```python
from build123d import *

# Parameters (mm, degrees)
F1_DEPTH = 20
F0_W     = 4
F0_H     = 2.9398608957
F2_DEPTH = 58
F4_DEPTH = 4
F5_DEPTH = 20
F7_DEPTH = 9


# Not quite as in the source:
# - a feature names something its author has since deleted; it is built from what else it names


with BuildPart() as f1:
    # F0 (on Top) → F1 (new body)
    with BuildSketch(Plane.XY):
        with BuildLine():
            Line((0, 13.7), (-25, 13.7))
            Line((-25, 13.7), (-25, -6))
            Line((-25, -6), (-12.3162494291, -6))
            ThreePointArc((-12.3162494291, -6), (-11.6165829744, 7.2625753008), (0, 13.7))
        make_face()
    extrude(amount=F1_DEPTH)



with BuildPart() as f1b:
    # F0 (on Top) → F1, piece 2 (new body)
    with BuildSketch(Plane.XY):
        with BuildLine():
            Line((25, 13.7), (0, 13.7))
            ThreePointArc((0, 13.7), (9.6873629023, 9.6873629023), (13.7, 0))
            ThreePointArc((13.7, 0), (13.3495808395, -3.0787483513), (12.3162494291, -6))
            Line((12.3162494291, -6), (25, -6))
            Line((25, -6), (25, 13.7))
        make_face()
    extrude(amount=F1_DEPTH)


with BuildPart() as f1_1:
    add(f1.part)

    add(f1b.part)  # F2 merges F1b
    # F0 (on Top) → F2 (join)
    with BuildSketch(Plane.XY):
        with BuildLine():
            ThreePointArc((13.7, 0), (9.6873629023, 9.6873629023), (0, 13.7))
            ThreePointArc((0, 13.7), (-11.6165829744, 7.2625753008), (-12.3162494291, -6))
            Line((-12.3162494291, -6), (-7.6216796049, -6))
            ThreePointArc((-7.6216796049, -6), (-3.1748785672, 9.1657048875), (9.7, 0))
            ThreePointArc((9.7, 0), (9.1657048875, -3.1748785672), (7.6216796049, -6))
            Line((7.6216796049, -6), (12.3162494291, -6))
            ThreePointArc((12.3162494291, -6), (13.3495808395, -3.0787483513), (13.7, 0))
        make_face()
        with BuildLine():
            Line((-7.6216796049, -6), (-12.3162494291, -6))
            ThreePointArc((-12.3162494291, -6), (-9.0959869464, -10.244658192), (-4.5, -12.9398608957))
            ThreePointArc((-4.5, -12.9398608957), (-2.5280436601, -13.4647315329), (-0.5, -13.6908728721))
            Line((-0.5, -13.6908728721), (-0.5, -9.6871048306))
            ThreePointArc((-0.5, -9.6871048306), (-4.4597203286, -8.6139941137), (-7.6216796049, -6))
        make_face()
        with BuildLine():
            ThreePointArc((4.5, -12.9398608957), (9.0959869464, -10.244658192), (12.3162494291, -6))
            Line((12.3162494291, -6), (7.6216796049, -6))
            ThreePointArc((7.6216796049, -6), (4.4597203286, -8.6139941137), (0.5, -9.6871048306))
            Line((0.5, -9.6871048306), (0.5, -13.6908728721))
            ThreePointArc((0.5, -13.6908728721), (2.5280436601, -13.4647315329), (4.5, -12.9398608957))
        make_face()
        with Locations((2.5, -15.4699304478)):
            Rectangle(F0_W, F0_H)
        with BuildLine():
            Line((4.5, -14), (4.5, -12.9398608957))
            ThreePointArc((4.5, -12.9398608957), (2.5280436601, -13.4647315329), (0.5, -13.6908728721))
            Line((0.5, -13.6908728721), (0.5, -14))
            Line((0.5, -14), (4.5, -14))
        make_face()
        with BuildLine():
            ThreePointArc((-0.5, -13.6908728721), (-2.5280436601, -13.4647315329), (-4.5, -12.9398608957))
            Line((-4.5, -12.9398608957), (-4.5, -14))
            Line((-4.5, -14), (-0.5, -14))
            Line((-0.5, -14), (-0.5, -13.6908728721))
        make_face()
        with Locations((-2.5, -15.4699304478)):
            Rectangle(F0_W, F0_H)
    extrude(amount=F2_DEPTH)

    # F3 (on face) → F4 (cut)
    with BuildSketch(Plane.XZ.offset(6)):
        with BuildLine():
            ThreePointArc((-21.3581247146, 10), (-18.6581247146, 12.7), (-15.9581247146, 10))
            Line((-15.9581247146, 10), (-13.4831247146, 10))
            ThreePointArc((-13.4831247146, 10), (-18.6581247146, 15.175), (-23.8331247146, 10))
            Line((-23.8331247146, 10), (-21.3581247146, 10))
        make_face()
        with BuildLine():
            Line((-13.4831247146, 10), (-15.9581247146, 10))
            ThreePointArc((-15.9581247146, 10), (-18.6581247146, 7.3), (-21.3581247146, 10))
            Line((-21.3581247146, 10), (-23.8331247146, 10))
            ThreePointArc((-23.8331247146, 10), (-18.6581247146, 4.825), (-13.4831247146, 10))
        make_face()
        with BuildLine():
            ThreePointArc((23.8331247146, 10), (18.6581247146, 15.175), (13.4831247146, 10))
            Line((13.4831247146, 10), (15.9581247146, 10))
            ThreePointArc((15.9581247146, 10), (18.6581247146, 12.7), (21.3581247146, 10))
            Line((21.3581247146, 10), (23.8331247146, 10))
        make_face()
        with BuildLine():
            Line((15.9581247146, 10), (13.4831247146, 10))
            ThreePointArc((13.4831247146, 10), (18.6581247146, 4.825), (23.8331247146, 10))
            Line((23.8331247146, 10), (21.3581247146, 10))
            ThreePointArc((21.3581247146, 10), (18.6581247146, 7.3), (15.9581247146, 10))
        make_face()
    extrude(amount=-F4_DEPTH, mode=Mode.SUBTRACT)

    # F5 (cut): faces of the model
    f5_faces = [f1_1.faces().sort_by_distance(p)[0] for p in [
        (-18.6581247146, -6, 10),
        (18.6581247146, -6, 10),
    ]]
    extrude(f5_faces, amount=-F5_DEPTH, mode=Mode.SUBTRACT)

    # F6 (on face) → F7 (cut)
    with BuildSketch(Plane(origin=(-4.5, 0, 0), x_dir=(0, -1, 0), z_dir=(-1, 0, 0))):
        with BuildLine():
            ThreePointArc((16.4898608957, 46.45), (16.0358764065, 47.5460155108), (14.9398608957, 48))
            Line((14.9398608957, 48), (14.9398608957, 44.9))
            ThreePointArc((14.9398608957, 44.9), (16.0358764065, 45.3539844892), (16.4898608957, 46.45))
        make_face()
        with BuildLine():
            ThreePointArc((16.4898608957, 11.55), (16.0358764065, 12.6460155108), (14.9398608957, 13.1))
            Line((14.9398608957, 13.1), (14.9398608957, 10))
            ThreePointArc((14.9398608957, 10), (16.0358764065, 10.4539844892), (16.4898608957, 11.55))
        make_face()
        with BuildLine():
            Line((14.9398608957, 10), (14.9398608957, 13.1))
            ThreePointArc((14.9398608957, 13.1), (13.3898608957, 11.55), (14.9398608957, 10))
        make_face()
        with BuildLine():
            ThreePointArc((16.4898608957, 29), (16.0358764065, 30.0960155108), (14.9398608957, 30.55))
            Line((14.9398608957, 30.55), (14.9398608957, 29))
            Line((14.9398608957, 29), (16.4898608957, 29))
        make_face()
        with BuildLine():
            Line((14.9398608957, 29), (14.9398608957, 30.55))
            ThreePointArc((14.9398608957, 30.55), (13.3898608957, 29), (14.9398608957, 27.45))
            Line((14.9398608957, 27.45), (14.9398608957, 29))
        make_face()
        with BuildLine():
            Line((14.9398608957, 44.9), (14.9398608957, 48))
            ThreePointArc((14.9398608957, 48), (13.3898608957, 46.45), (14.9398608957, 44.9))
        make_face()
        with BuildLine():
            Line((16.4898608957, 29), (14.9398608957, 29))
            Line((14.9398608957, 29), (14.9398608957, 27.45))
            ThreePointArc((14.9398608957, 27.45), (16.0358764065, 27.9039844892), (16.4898608957, 29))
        make_face()
    extrude(amount=-F7_DEPTH, mode=Mode.SUBTRACT)


solid = f1_1.part
```
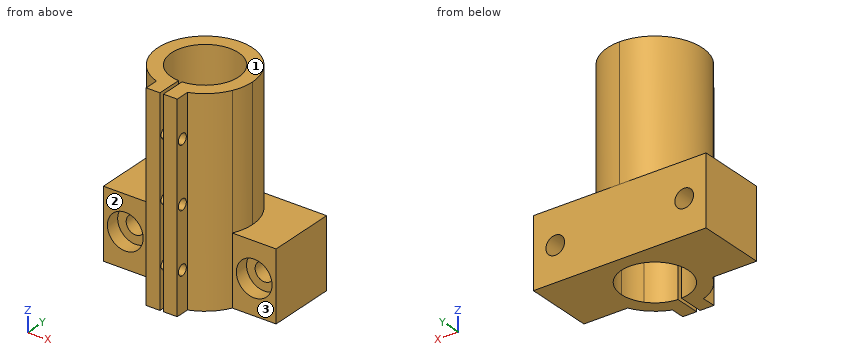
Here's how the part is built. I have some questions about the finished solid (model axes, mm). Face numbers are marked on the shaded views. A direction names the side the tool comes from. Give positions to 0.01 mm unless a question says otherwise; leave off trailing zeros. Order: outer loops, then holes, each group sorted by start corner. A loop starts at its lowest first (then second) coordinate and runs counter-clockwise, first axis right, second up. Notation, with made-up numbers: (63.5, 37.5) - (117.5, 37.5) arc R14 cw to (117.5, 54.5) - close; hole circle Ø9 at (32.5, 50.5). An arc over 180 degrees is marked (long way). Answer as a JSON object with one key per item and string values. Group by question number.
Item 1: For P1, Ø8.5, axis at x = -21, z = 10.5, coming from the -Y side; P2, Ø4.5, axis at y = -15.5, z = 36, coming from the +X side; P3, Ø3, axis at x = 20.5, z = 12.5, coming from the -Y side, each with a flat end and sliding along its axis, tell me the tip position at first contact or that it passes through.
Item 2: If we section it at C-C on x = 20: Please give me the cut outline in (y, z), and give its area (3 significant figures).
Item 3: Which directions (+Z, -Z, +X, -X, +Y, -Y) give clear straight access to the entire face, cutting with the end or side of a thin tool? Please do the marked faces 1, 2 and 3.
Item 4: If we section it at D-D on y = 11.5: Please give me the cut outline in (x, z).
Item 5: If we section it at B-B on z = 38.5: Please give me the cut outline in (x, y), and give its area (3 significant figures).
Item 6: If we section it at A-A on y = 2: Please give me the cut outline in (x, z), and give its area (3 significant figures).
Item 7: Please list where these lines run through material, in increasing order: probe 1 along X at (y, z) = (-6, 49.5); probe 2 along X at (y, z) = (3.25, 10); probe 3 along X at (y, z) = (1.25, 10).
Result set:
{
 "1": {"P1": "y = -6", "P2": "x = 4.5", "P3": "y = -2"},
 "2": {"outline": "(-6, 0) - (13.7, 0) - (13.7, 7.66) - (-2, 7.66) - (-2, 5) - (-6, 5) - close; (-6, 15) - (-2, 15) - (-2, 12.34) - (13.7, 12.34) - (13.7, 20) - (-6, 20) - close", "area": "280 mm²"},
 "3": {"face 1": "+Z, +X, -X, +Y, -Y", "face 2": "+Z, -Z, -X, -Y", "face 3": "+Z, -Z, +X, -Y"},
 "4": {"outline": "(-25, 0) - (25, 0) - (25, 20) - (7.45, 20) - (7.45, 58) - (-7.45, 58) - (-7.45, 20) - (-25, 20) - close; hole circle Ø5.4 at (-18.66, 10); hole circle Ø5.4 at (18.66, 10)"},
 "5": {"outline": "(-4.5, -16.94) - (-0.5, -16.94) - (-0.5, -9.69) arc R9.7 cw (long way) to (0.5, -9.69) - (0.5, -16.94) - (4.5, -16.94) - (4.5, -12.94) arc R13.7 ccw (long way) to (-4.5, -12.94) - close", "area": "318 mm²"},
 "6": {"outline": "(-25, 0) - (-9.49, 0) - (-9.49, 58) - (-13.55, 58) - (-13.55, 20) - (-25, 20) - close; (9.49, 0) - (25, 0) - (25, 20) - (13.55, 20) - (13.55, 58) - (9.49, 58) - close; hole circle Ø5.4 at (-18.66, 10); hole circle Ø5.4 at (18.66, 10)", "area": "883 mm²"},
 "7": {"probe 1": "-12.32 to -7.62, 7.62 to 12.32", "probe 2": "-25 to -21.36, -15.96 to -9.14, 9.14 to 15.96, 21.36 to 25", "probe 3": "-25 to -21.36, -15.96 to -9.62, 9.62 to 15.96, 21.36 to 25"}
}
